```python
from build123d import *

# Parameters (mm, degrees)
SKETCH1_W                                    = 500
SKETCH1_H                                    = 592
BOSS_EXTRUDE1_DEPTH                          = 4
CSK_FOR_M6_HEX_SOCKET_COUNTERSUNK_CA_2_COUNT = 2
CSK_FOR_M6_HEX_SOCKET_COUNTERSUNK_CA_2_PITCH = 460
CSK_FOR_M6_HEX_SOCKET_COUNTERSUNK_CA_3_COUNT = 2
CSK_FOR_M6_HEX_SOCKET_COUNTERSUNK_CA_3_PITCH = 272.73430294
CSK_FOR_M6_HEX_SOCKET_COUNTERSUNK_CA_4_COUNT = 2
CSK_FOR_M6_HEX_SOCKET_COUNTERSUNK_CA_4_PITCH = 356.207804519
CSK_FOR_M6_HEX_SOCKET_COUNTERSUNK_CA_5_COUNT = 2
CSK_FOR_M6_HEX_SOCKET_COUNTERSUNK_CA_5_PITCH = 517.28522113
CSK_FOR_M6_HEX_SOCKET_COUNTERSUNK_CA_6_COUNT = 2
CSK_FOR_M6_HEX_SOCKET_COUNTERSUNK_CA_6_PITCH = 521.536192416
CSK_FOR_M6_HEX_SOCKET_COUNTERSUNK_CA_7_COUNT = 2
CSK_FOR_M6_HEX_SOCKET_COUNTERSUNK_CA_7_PITCH = 362.35341864
CSK_FOR_M6_HEX_SOCKET_COUNTERSUNK_CA_8_COUNT = 2
CSK_FOR_M6_HEX_SOCKET_COUNTERSUNK_CA_8_PITCH = 280.713376952


with BuildPart() as part:
    # Sketch1 → Boss-Extrude1 (new body)
    with BuildSketch(Plane.XY):
        Rectangle(SKETCH1_W, SKETCH1_H)
    extrude(amount=BOSS_EXTRUDE1_DEPTH)

    # Sketch4 → CSK for M6 Hex Socket Countersunk Cap Screw1 (revolve, cut)
    with BuildSketch(Plane(origin=(-230, -4, 4), x_dir=(0, -1, 0), z_dir=(1, 0, 0))):
        Polygon((0, 0), (0, 4), (3.3, 4), (3.3, 3.42), (6.72, 0), align=None)
    csk_for_m6_hex_socket_countersunk_cap_sc = revolve(axis=Axis((-230, -4, 10.35), (0, 0, -1)), mode=Mode.SUBTRACT)

    # CSK for M6 Hex Socket Countersunk Ca 2: CSK for M6 Hex Socket Countersunk Cap Screw1 ×2
    with Locations(*[(i * CSK_FOR_M6_HEX_SOCKET_COUNTERSUNK_CA_2_PITCH, 0, 0) for i in range(1, CSK_FOR_M6_HEX_SOCKET_COUNTERSUNK_CA_2_COUNT)]):
        add(csk_for_m6_hex_socket_countersunk_cap_sc, mode=Mode.SUBTRACT)

    # CSK for M6 Hex Socket Countersunk Ca 3: CSK for M6 Hex Socket Countersunk Cap Screw1 ×2
    with Locations(*[Vector(0.07333144303605385, -0.9973076252903365, 0) * (i * CSK_FOR_M6_HEX_SOCKET_COUNTERSUNK_CA_3_PITCH) for i in range(1, CSK_FOR_M6_HEX_SOCKET_COUNTERSUNK_CA_3_COUNT)]):
        add(csk_for_m6_hex_socket_countersunk_cap_sc, mode=Mode.SUBTRACT)

    # CSK for M6 Hex Socket Countersunk Ca 4: CSK for M6 Hex Socket Countersunk Cap Screw1 ×2
    with Locations(*[Vector(0.6456905129038378, -0.7635992152601906, 0) * (i * CSK_FOR_M6_HEX_SOCKET_COUNTERSUNK_CA_4_PITCH) for i in range(1, CSK_FOR_M6_HEX_SOCKET_COUNTERSUNK_CA_4_COUNT)]):
        add(csk_for_m6_hex_socket_countersunk_cap_sc, mode=Mode.SUBTRACT)

    # CSK for M6 Hex Socket Countersunk Ca 5: CSK for M6 Hex Socket Countersunk Cap Screw1 ×2
    with Locations(*[Vector(0.8505945695460384, -0.525822097537551, 0) * (i * CSK_FOR_M6_HEX_SOCKET_COUNTERSUNK_CA_5_PITCH) for i in range(1, CSK_FOR_M6_HEX_SOCKET_COUNTERSUNK_CA_5_COUNT)]):
        add(csk_for_m6_hex_socket_countersunk_cap_sc, mode=Mode.SUBTRACT)

    # CSK for M6 Hex Socket Countersunk Ca 6: CSK for M6 Hex Socket Countersunk Cap Screw1 ×2
    with Locations(*[Vector(0.8436614877321075, 0.5368754921931593, 0) * (i * CSK_FOR_M6_HEX_SOCKET_COUNTERSUNK_CA_6_PITCH) for i in range(1, CSK_FOR_M6_HEX_SOCKET_COUNTERSUNK_CA_6_COUNT)]):
        add(csk_for_m6_hex_socket_countersunk_cap_sc, mode=Mode.SUBTRACT)

    # CSK for M6 Hex Socket Countersunk Ca 7: CSK for M6 Hex Socket Countersunk Cap Screw1 ×2
    with Locations(*[Vector(0.6347394233600139, 0.7727262545252344, 0) * (i * CSK_FOR_M6_HEX_SOCKET_COUNTERSUNK_CA_7_PITCH) for i in range(1, CSK_FOR_M6_HEX_SOCKET_COUNTERSUNK_CA_7_COUNT)]):
        add(csk_for_m6_hex_socket_countersunk_cap_sc, mode=Mode.SUBTRACT)

    # CSK for M6 Hex Socket Countersunk Ca 8: CSK for M6 Hex Socket Countersunk Cap Screw1 ×2
    with Locations(*[Vector(0.07124704998790936, 0.9974586998307351, 0) * (i * CSK_FOR_M6_HEX_SOCKET_COUNTERSUNK_CA_8_PITCH) for i in range(1, CSK_FOR_M6_HEX_SOCKET_COUNTERSUNK_CA_8_COUNT)]):
        add(csk_for_m6_hex_socket_countersunk_cap_sc, mode=Mode.SUBTRACT)


solid = part.part
```
Build history of the part. All positions in model axes, mm. Give positions to 0.01 mm unless a question says otherwise; leave off trailing zeros. Use a Markdown table: item, result.
(1) Drop flat-ended pins along their axis: pin 1 Ø8.5 at (x, y) = (-210, 276) entering from +Z; pin 2 Ø10.5 at (x, y) = (210, 276) entering from +Z. Give the stop position or say it passes through.
Taken from the geometry:
| item | result |
|---|---|
| pin 1 | z = 1.53 |
| pin 2 | z = 2.53 |
(2) Pull direction Y, two halves, no side cores. Call faces 1 (the face through (-3, 4, 0)), 2 (the face through (-213.48, 276.46, 0.79)), 3 (the face through (207.63, 278.59, 0.79)): +Y half, -Y half, draft (parallel to the pull), parting line (faces both ways), or undercut.
Taken from the geometry:
| item | result |
|---|---|
| face 1 | draft |
| face 2 | undercut |
| face 3 | undercut |
(3) Wall check: line 1 along X through (y, z) = (276, 0.15); line 2 along Y through (x, z) = (210, 0.35); line 3 along X through (y, z) = (-4, 0.4). Give the ranges that are in metal, low to high.
Taken from the geometry:
| item | result |
|---|---|
| line 1 | -250 to -213.3, -206.7 to -3.3, 3.3 to 206.7, 213.3 to 250 |
| line 2 | -296 to -279.3, -272.7 to 272.7, 279.3 to 296 |
| line 3 | -250 to -233.3, -226.7 to 226.7, 233.3 to 250 |
